```python
from build123d import *

# Parameters (mm, degrees)
SKETCH_1_W          = 29
SKETCH_1_H          = 82
EXTRUDE_1_DEPTH     = 18
CHAMFER_1_SIZE      = 3
FILLET_1_R          = 3
SKETCH_2_R          = 3
CUT_EXTRUDE_1_DEPTH = 5
CUT_EXTRUDE_START   = -5
SKETCH_3_R          = 3
CUT_EXTRUDE_2_DEPTH = 5


with BuildPart() as part:
    # 草图1 → 凸台-拉伸1 (new body)
    with BuildSketch(Plane.XY):
        with Locations((-13.005076144, -29.675385896)):
            Rectangle(SKETCH_1_W, SKETCH_1_H)
        with BuildLine():
            Line((-3.505076144, 5.324614104), (-3.505076144, -64.675385896))
            Line((-3.505076144, -64.675385896), (-17.505076144, -64.675385896))
            ThreePointArc((-17.505076144, -64.675385896), (-20.005076144, -62.175385896), (-17.505076144, -59.675385896))
            Line((-17.505076144, -59.675385896), (-17.505076144, -54.675385896))
            ThreePointArc((-17.505076144, -54.675385896), (-19.005076144, -53.175385896), (-17.505076144, -51.675385896))
            Line((-17.505076144, -51.675385896), (-17.505076144, -7.675385896))
            ThreePointArc((-17.505076144, -7.675385896), (-19.005076144, -6.175385896), (-17.505076144, -4.675385896))
            Line((-17.505076144, -4.675385896), (-17.505076144, 0.324614104))
            ThreePointArc((-17.505076144, 0.324614104), (-20.005076144, 2.824614104), (-17.505076144, 5.324614104))
            Line((-17.505076144, 5.324614104), (-3.505076144, 5.324614104))
        make_face(mode=Mode.SUBTRACT)
    extrude(amount=EXTRUDE_1_DEPTH)

    # 倒角1
    chamfer_1_edges = [part.edges().sort_by_distance(p)[0] for p in [
        (1.494923856, 11.324614104, 9),
        (1.494923856, -70.675385896, 9),
        (-27.505076144, -70.675385896, 9),
        (-27.505076144, 11.324614104, 9),
    ]]
    chamfer(chamfer_1_edges, length=CHAMFER_1_SIZE)

    # 圆角1
    fillet_1_edges = [part.edges().sort_by_distance(p)[0] for p in [
        (-27.505076144, -29.675385896, 0),
        (-27.505076144, -29.675385896, 18),
        (1.494923856, -29.675385896, 0),
        (1.494923856, -29.675385896, 18),
    ]]
    fillet(fillet_1_edges, radius=FILLET_1_R)

    # 草图2 → 切除-拉伸1 (cut)
    with BuildSketch(Plane.XZ.offset(70.675385896)):
        with Locations(Location((-12.505076144, 9, 0), (0, 0, 270))):
            Circle(SKETCH_2_R)
    extrude(amount=-CUT_EXTRUDE_1_DEPTH, mode=Mode.SUBTRACT)

    # 草图3 → 切除-拉伸2 (cut)
    with BuildSketch(Plane(origin=(0, 11.324614104, 0), x_dir=(1, 0, 0), z_dir=(0, 1, 0)).offset(CUT_EXTRUDE_START)):
        with Locations(Location((-12.505076144, -9, 0), (0, 0, 90))):
            Circle(SKETCH_3_R)
    extrude(amount=CUT_EXTRUDE_2_DEPTH, mode=Mode.SUBTRACT)


solid = part.part
```
Could you check a few things on this model? Use its own coordinates, in mm. A direction names the side the tool comes from. Give positions to 0.01 mm unless a question says otherwise; leave off trailing zeros. Loops run counter-clockwise (first coordinate to the right, second up) from the corner with the lowest first, then second, coordinate; pieces in that order, holes last. Notation, with made-up numbers: (-28.75, 74.5) -> (21.25, 74.5) arc R36 cw to (21.25, 110.5) -> close; hole circle Ø8 at (79.5, 11.25). An arc over 180 degrees is marked (long way). Put each result on its own line as item: value.
(1) Imagine slicing it at C-C on x = -16.25. Write out the boundary of the cut face in (y, z).
Computed:
outline: (-70.68, 0) -> (-64.68, 0) -> (-64.68, 18) -> (-70.68, 18) -> close; (5.32, 0) -> (11.32, 0) -> (11.32, 18) -> (5.32, 18) -> close
(2) For faces 1 (the face through (-10, -64.675, 9)), 2 (the face through (0.02, -69.15, 8.87)), which set-ups out of +Z, -Z, +X, -X, +Y, -Y let a thin tool reach every point of the face, with its end or its side?
Computed:
face 1: +Z, -Z
face 2: +Z, -Z, +X, -Y
(3) I'm going to push flat-ended pins straight in: pin 1 Ø5.5 at (x, z) = (-12.51, 9) entering from +Y; pin 2 Ø3 at (x, z) = (-13.5, 9.5) entering from -Y. Where does each tip first touch, or does it pass through?
Computed:
pin 1: y = 6.32
pin 2: y = -65.68
(4) Imagine slicing it at B-B on z = 9. Write out the boundary of the cut face in (x, y).
Computed:
outline: (-27.51, -67.68) -> (-24.51, -70.68) -> (-15.51, -70.68) -> (-15.51, -65.68) -> (-9.51, -65.68) -> (-9.51, -70.68) -> (-1.51, -70.68) -> (1.49, -67.68) -> (1.49, 8.32) -> (-1.51, 11.32) -> (-9.51, 11.32) -> (-9.51, 6.32) -> (-15.51, 6.32) -> (-15.51, 11.32) -> (-24.51, 11.32) -> (-27.51, 8.32) -> close; hole (-17.51, -64.68) -> (-3.51, -64.68) -> (-3.51, 5.32) -> (-17.51, 5.32) arc R2.5 ccw to (-17.51, 0.32) -> (-17.51, -4.68) arc R1.5 ccw to (-17.51, -7.68) -> (-17.51, -51.68) arc R1.5 ccw to (-17.51, -54.68) -> (-17.51, -59.68) arc R2.5 ccw to start
(5) Imagine slicing it at A-A on y = -45.5. Write out the boundary of the cut face in (x, z), plus the area to 3 significant figures.
Computed:
outline: (-27.51, 3) arc R3 ccw to (-24.51, 0) -> (-17.51, 0) -> (-17.51, 18) -> (-24.51, 18) arc R3 ccw to (-27.51, 15) -> close; (-3.51, 0) -> (-1.51, 0) arc R3 ccw to (1.49, 3) -> (1.49, 15) arc R3 ccw to (-1.51, 18) -> (-3.51, 18) -> close
area: 262 mm^2
(6) Imagine slicing it at D-D on z = 14. Write out the boundary of the cut face in (x, y), plus the area to 3 significant figures.
Computed:
outline: (-27.51, -67.68) -> (-24.51, -70.68) -> (-1.51, -70.68) -> (1.49, -67.68) -> (1.49, 8.32) -> (-1.51, 11.32) -> (-24.51, 11.32) -> (-27.51, 8.32) -> close; hole (-17.51, -64.68) -> (-3.51, -64.68) -> (-3.51, 5.32) -> (-17.51, 5.32) arc R2.5 ccw to (-17.51, 0.32) -> (-17.51, -4.68) arc R1.5 ccw to (-17.51, -7.68) -> (-17.51, -51.68) arc R1.5 ccw to (-17.51, -54.68) -> (-17.51, -59.68) arc R2.5 ccw to start
area: 1,350 mm^2
(7) Thinking about a two-plate mould opening in Z: for faces 3 (the face through (0.02, 9.8, 8.87)), 4 (the face through (-26.65, -29.1, 17.1)), 5 (the face through (-9.53, -68.21, 9.39)), 6 (the face through (-13, 6.325, 9)), which applies, pulls with the +Z half, pulls with the -Z half, needs draft (parallel to the pull), parting line crosses it, or undercut?
Computed:
face 3: needs draft
face 4: pulls with the +Z half
face 5: undercut
face 6: undercut
(8) Please list where these lines run through material, in increasing order: probe 1 along X at (y, z) = (-59, 10); probe 2 along X at (y, z) = (-67.3, 9); probe 3 along Y at (x, z) = (-14.5, 5.25). Write a range as [from, to].
Computed:
probe 1: [-27.51, -17.51], [-3.51, 1.49]
probe 2: [-27.51, -15.51], [-9.51, 1.49]
probe 3: [-70.68, -64.68], [5.32, 11.32]
